The model under review builds one solid part; all positions refer to its coordinate system, in mm. Give positions to 0.01 mm unless a question says otherwise; leave off trailing zeros. Loops run counter-clockwise (first coordinate to the right, second up) from the corner with the lowest first, then second, coordinate; pieces in that order, holes last. Notation, with made-up numbers: M 55.25,-37 L 63.25,-37 A23 ccw 63.25,-29 Z; hole C 83,-32 d8. An arc over 180 degrees is marked long. Write item = value, one per line. Start each with the question number.
1. Draft analysis for pull direction Y (two halves, no side actions). For faces 1 (the face through (-238, -124, 4.762)), 2 (the face through (-385.503, -180.713, 2.348)), state which applies: pulls with the +Y half, pulls with the -Y half, needs draft (parallel to the pull), parting line crosses it, or undercut.
2. For pin 1 (2.5 mm diameter, centred on x = 2.5, z = 3.5, fed in from +Y); pin 2 (2.5 mm diameter, centred on y = -69.5, z = 2, fed in from +X), all flat-tipped, find the tip position at first contact; note any pin that passes through.
3. We need section D-D on x = -357.5. Give the boundary of the cut face in (y, z), then the cut area to 3 significant figures.
4. We need section C-C on y = -280. Give the boundary of the cut face in (x, z).
5. We need section A-A on x = -32.5. Give the boundary of the cut face in (y, z).
6. We need section B-B on z = 2.9. Give the boundary of the cut face in (x, y).
7. Wall thickness on line 1 along Y through (x, z) = (-128.5, 1.9); line 2 along X through (y, z) = (-216.5, 3.8); line 3 along X through (y, z) = (15, 3.65): over which ranges is each line inside the solid? List them lowest first. Write a range as from..to.
Autodesk Inventor part; units mm, degrees
ref_plane "YZ Plane" through (0, 0, 0) normal (1, 0, 0) x (0, 1, 0)
ref_plane "XZ Plane" through (0, 0, 0) normal (0, 1, 0) x (-1, 0, 0)
ref_plane "XY Plane" through (0, 0, 0) normal (0, 0, 1) x (1, 0, 0)
ref_plane "Work Plane1" through (0, 0, 0) normal (0, 0, 1) x (1, 0, 0)
sketch "Sketch2" plane through (0, 0, 0) normal (0, 0, 1) x (1, 0, 0)
  line L0 (5.0006, 57.6014) -> (-474.9994, 57.6014)
  line L1 (-474.9994, 57.6014) -> (-474.9994, -309.9996)
  line L2 (-474.9994, -309.9996) -> (5.0006, -309.9996)
  line L3 (5.0006, -309.9996) -> (5.0006, 57.6014)
  line L4 (5.0006, -239.9996) -> (0.2381, -239.9996)
  line L5 (0.2381, -239.9996) -> (0.2381, -269.9996)
  line L6 (0.2381, -269.9996) -> (5.0006, -269.9996)
  line L7 (5.0006, -269.9996) -> (5.0006, -239.9996)
  line L8 (5.0006, -159.9996) -> (0.2381, -159.9996)
  line L9 (0.2381, -159.9996) -> (0.2381, -189.9996)
  line L10 (0.2381, -189.9996) -> (5.0006, -189.9996)
  line L11 (5.0006, -189.9996) -> (5.0006, -159.9996)
  line L12 (5.0006, 0.0004) -> (0.2381, 0.0004)
  line L13 (0.2381, 0.0004) -> (0.2381, -29.9996)
  line L14 (0.2381, -29.9996) -> (5.0006, -29.9996)
  line L15 (5.0006, -29.9996) -> (5.0006, 0.0004)
  line L16 (5.0006, -79.9996) -> (0.2381, -79.9996)
  line L17 (0.2381, -79.9996) -> (0.2381, -109.9996)
  line L18 (0.2381, -109.9996) -> (5.0006, -109.9996)
  line L19 (5.0006, -109.9996) -> (5.0006, -79.9996)
  line L20 (5.0006, 57.6014) -> (0.2381, 57.6014)
  line L21 (0.2381, 57.6014) -> (0.2381, -309.9996)
  line L22 (0.2381, -309.9996) -> (5.0006, -309.9996)
  line L23 (5.0006, -309.9996) -> (5.0006, 57.6014)
  line L24 (5.0006, 57.6014) -> (-474.9994, 57.6014)
  line L25 (-474.9994, 57.6014) -> (-474.9994, 54.6014)
  line L26 (-474.9994, 54.6014) -> (5.0006, 54.6014)
  line L27 (5.0006, 54.6014) -> (5.0006, 57.6014)
  line L28 (-474.9994, -309.9996) -> (5.0006, -309.9996)
  line L29 (5.0006, -309.9996) -> (5.0006, -306.9996)
  line L30 (5.0006, -306.9996) -> (-474.9994, -306.9996)
  line L31 (-474.9994, -306.9996) -> (-474.9994, -309.9996)
  line L32 (5.0006, -65.3986) -> (-474.9994, -65.3986)
  line L33 (-474.9994, -65.3986) -> (-474.9994, -75.3986)
  line L34 (-474.9994, -75.3986) -> (5.0006, -75.3986)
  line L35 (5.0006, -75.3986) -> (5.0006, -65.3986)
  line L36 (-474.9994, -65.3986) -> (-235.9994, -65.3986)
  line L37 (-235.9994, -65.3986) -> (-235.9994, -75.3986)
  line L38 (-235.9994, -75.3986) -> (-474.9994, -75.3986)
  line L39 (-474.9994, -75.3986) -> (-474.9994, -65.3986)
  circle A0 centre (-282.9994, -259.9996) radius 30
  circle A1 centre (-186.9994, -209.9996) radius 30
  circle A2 centre (-90.9994, -259.9996) radius 30
  circle A3 centre (-378.9994, -209.9996) radius 30
  point P0 (0, 0)
  point P1 (0.2381, -306.9996)
  point P2 (0.2381, -239.9996)
  point P3 (0.2381, 54.6014)
  point P4 (-235.9994, -65.3986)
  point P5 (0.2381, -65.3986)
  point P6 (0.2381, -75.3986)
  point P7 (-235.9994, -75.3986)
  dimension "d14" = 480
  dimension "d15" = 367.601
  dimension "d16" = 4.7625
  dimension "d17" = 30
  dimension "d18" = 4.7625
  dimension "d19" = 30
  dimension "d20" = 4.7625
  dimension "d21" = 30
  dimension "d22" = 4.7625
  dimension "d23" = 30
  dimension "d24" = 40
  dimension "d25" = 50
  dimension "d26" = 50
  dimension "d27" = 50
  dimension "d28" = 4.7625
  dimension "d29" = 367.601
  dimension "d30" = 3
  dimension "d31" = 3
  dimension "d34" = 480
  dimension "d35" = 10
  dimension "d36" = 123
  dimension "d37" = 239
  dimension "d38" = 10
  dimension "d39" = 60
  dimension "d40" = 60
  dimension "d41" = 60
  dimension "d42" = 60
  dimension "d43" = 50
  dimension "d45" = 50
  dimension "d46" = 100
  dimension "d47" = 100
  dimension "d48" = 96
  dimension "d49" = 96
  dimension "d50" = 96
  dimension "d51" = 96
extrude "Extrusion1" add sketch "Sketch2" along normal blind 4.7625 contours L21 L13 L32 L1 L26 | L3 L14 L13 L12 | L32 L37 L34 L1 | L34 L21 L17 L9 L5 L30 L1 | L3 L18 L17 L16 | L5 L4 L3 L6 | L3 L10 L9 L8
properties part number "leg 2" material "foam core"
Final values:
q1.face_1 = needs draft
q1.face_2 = undercut
q2.pin_1 = 0
q2.pin_2 = -236
q3.outline = M -307,0 L -230.92,0 L -230.92,4.76 L -307,4.76 Z; M -189.08,0 L 54.6,0 L 54.6,4.76 L -189.08,4.76 Z
q3.area = 1,520 mm²
q4.outline = M -475,0 L -305.36,0 L -305.36,4.76 L -475,4.76 Z; M -260.64,0 L -113.36,0 L -113.36,4.76 L -260.64,4.76 Z; M -68.64,0 L 0.24,0 L 0.24,4.76 L -68.64,4.76 Z
q5.outline = M -307,0 L -75.4,0 L -75.4,4.76 L -307,4.76 Z; M -65.4,0 L 54.6,0 L 54.6,4.76 L -65.4,4.76 Z
q6.outline = M -475,-307 L 0.24,-307 L 0.24,-270 L 5,-270 L 5,-240 L 0.24,-240 L 0.24,-190 L 5,-190 L 5,-160 L 0.24,-160 L 0.24,-110 L 5,-110 L 5,-80 L 0.24,-80 L 0.24,-75.4 L -236,-75.4 L -236,-65.4 L 0.24,-65.4 L 0.24,-30 L 5,-30 L 5,0 L 0.24,0 L 0.24,54.6 L -475,54.6 Z; hole C -379,-210 d60; hole C -283,-260 d60; hole C -187,-210 d60; hole C -91,-260 d60
q7.line_1 = -307..-75.4, -65.4..54.6
q7.line_2 = -475..-408.29, -349.71..-216.29, -157.71..0.24
q7.line_3 = -475..0.24
